Read the model definition and answer for the solid it produces. Units are mm, in the model's axes. Face numbers are marked on the shaded views. A direction names the side the tool comes from. Round coordinates to 2 decimals unless told otherwise and drop trailing zeros. Write each loop counter-clockwise with the first axis right and the second up, starting at its lowest first coordinate (ties: lowest second). Pieces come first, ordered by that corner, then holes.
from build123d import *

# Parameters (mm, degrees)
CUT_EXTRUDE5_DEPTH      = 6
CUT_EXTRUDE5_DEPTH_BACK = 6
SKETCH3_R               = 3
BOSS_EXTRUDE1_DEPTH     = 7
SKETCH4_R               = 2
BOSS_EXTRUDE2_DEPTH     = 1


with BuildPart() as part:
    # Sketch1 → Revolve1 (revolve)
    with BuildSketch(Plane.XY):
        with BuildLine():
            Line((0, -1), (5, -1))
            Line((5, -1), (5, 1))
            ThreePointArc((5, 1), (2.837274331, 2.970139283), (0, 3.68337521))
            Line((0, 3.68337521), (0, -1))
        make_face()
    revolve(axis=Axis((0, 3.68337521, 0), (0, -1, 0)))

    # Sketch2 → Cut-Extrude5 (cut, two sides)
    with BuildSketch(Plane.XY) as cut_extrude5_sk:
        Polygon((-1, 28.719638355), (-1, 3.599454993), (-1, 1.599454993), (1, 1.599454993), (1, 3.599454993), (1, 28.719638355), (1, 78.960005081), (-1, 78.960005081), align=None)
    extrude(amount=CUT_EXTRUDE5_DEPTH, mode=Mode.SUBTRACT)
    extrude(cut_extrude5_sk.sketch, amount=-CUT_EXTRUDE5_DEPTH_BACK, mode=Mode.SUBTRACT)

    # Sketch3 → Boss-Extrude1 (add)
    with BuildSketch(Plane.XZ.offset(1)):
        Circle(SKETCH3_R)
    extrude(amount=BOSS_EXTRUDE1_DEPTH)

    # Sketch4 → Boss-Extrude2 (add)
    with BuildSketch(Plane.XZ.offset(8)):
        Circle(SKETCH4_R)
    extrude(amount=BOSS_EXTRUDE2_DEPTH)


solid = part.part
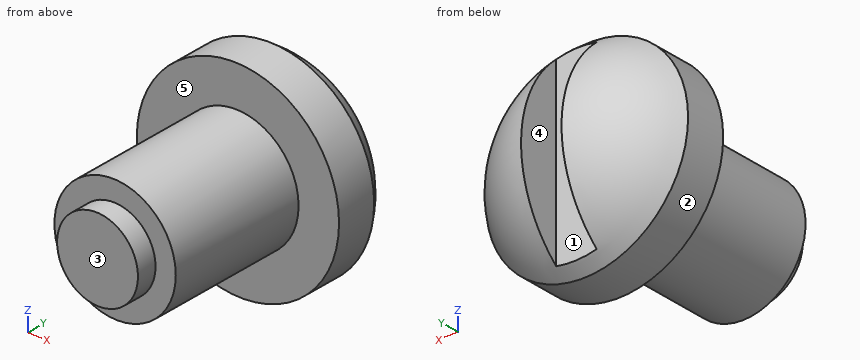
Q1. Section C-C (y = 2.25) is taken. Determine the outline of the cut face in (x, z), then the cut area to 3 significant figures.
Verdict:
outline: (-1, -3.76) - (-1, 3.76) arc R3.89 ccw to start; (1, -3.76) arc R3.89 ccw to (1, 3.76) - close
area: 32.2 mm2
Q2. Section B-B (z = 0) is taken. Determine the outline of the cut face in (x, y).
Verdict:
outline: (-5, -1) - (-3, -1) - (-3, -8) - (-2, -8) - (-2, -9) - (2, -9) - (2, -8) - (3, -8) - (3, -1) - (5, -1) - (5, 1) arc R6 ccw to (1, 3.6) - (1, 1.6) - (-1, 1.6) - (-1, 3.6) arc R6 ccw to (-5, 1) - close
Q3. Which of the six approach directions +Z, -Z, +X, -X, +Y, -Y give full straight-line access (tool end or side, diameter ignored) to the marked faces 4 and 5?
Verdict:
face 4: +Z, -Z, +Y
face 5: -Y
Q4. Section A-A (x = 0) is taken. Determine the outline of the cut face in (y, z), then the cut area to 3 significant figures.
Verdict:
outline: (-9, -2) - (-8, -2) - (-8, -3) - (-1, -3) - (-1, -5) - (1, -5) arc R6 ccw to (1.6, -4.55) - (1.6, 4.55) arc R6 ccw to (1, 5) - (-1, 5) - (-1, 3) - (-8, 3) - (-8, 2) - (-9, 2) - close
area: 71.7 mm2
Q5. Section D-D (y = -5.25) is taken. Determine the outline of the cut face in (x, z).
Verdict:
outline: circle Ø6 at (0, 0)
Q6. Straight lines are drawn through the part: probe 1 along Y at (x, z) = (0.25, 0.5); probe 2 along Y at (x, z) = (-0.5, 2); probe 3 along X at (y, z) = (2, 2.5). For each, find the intervals that lie inside material, in ascending order.
Verdict:
probe 1: y = -9 to 1.6
probe 2: y = -8 to 1.6
probe 3: x = -3.33 to -1, 1 to 3.33
Q7. Flat-ended cylindrical pins translate along their axes: pin 1 Ø1 at (y, z) = (2.5, 1.5) entering from +X; pin 2 Ø6 at (x, y) = (-3.5, -1.5) entering from -Z; pin 3 Ø2 at (y, z) = (-6.5, 2.5) entering from +X. Find the tip coordinate at first contact, or state that the pin passes through.
Verdict:
pin 1: stops at x = 3.92
pin 2: stops at z = -4.97
pin 3: stops at x = 2.6
Q8. Determine the mould class of the marked faces 1, 2 and 3 for opening direction X: pulls with the +X half, pulls with the -X half, needs draft (parallel to the pull), parting line crosses it, or undercut.
Verdict:
face 1: undercut
face 2: parting line crosses it
face 3: needs draft
